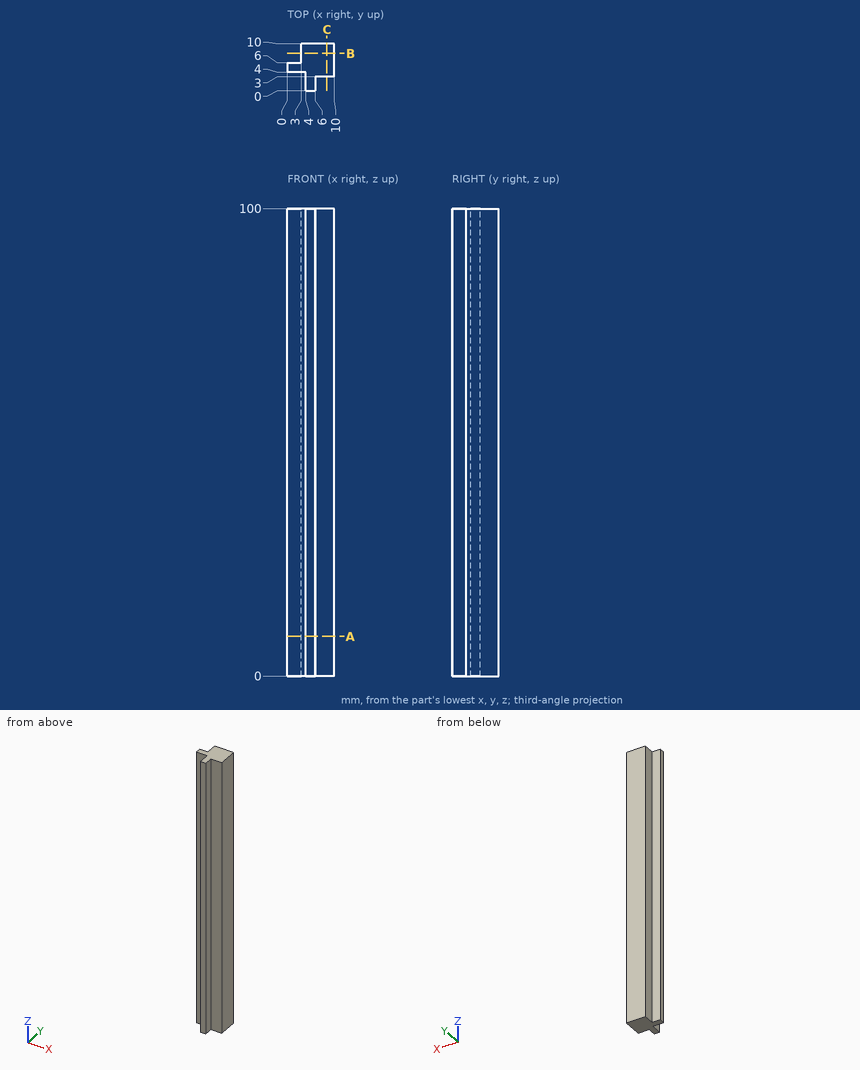
For this review, use the dimensioned drawing (mm, ordinates from the lowest corner) and the shaded views. Round coordinates to 2 decimals unless told otherwise and drop trailing zeros. Order: outer loops, then holes, each group sorted by start corner. A loop starts at its lowest first (then second) coordinate and runs counter-clockwise, first axis right, second up.
1) Consider section A-A (z = 8.5). State the section outline as (x, y) points.
The answers:
outline: (0, 4) - (4, 4) - (4, 0) - (6, 0) - (6, 3) - (10, 3) - (10, 10) - (3, 10) - (3, 6) - (0, 6) - close
2) Clearance check with flat-ended pins moving along their axes: pin 1 Ø1.5 at (x, y) = (3, 5) entering from -Z; pin 2 Ø1.5 at (x, z) = (1, 34.5) entering from +Y. State where each tip first meets the part, or that it passes through.
The answers:
pin 1: stops at z = 0
pin 2: stops at y = 6
3) For L1, parallel to X at y = 2.25, z = 82; L2, parallel to X at y = 9.5, z = 22; L3, parallel to Y at x = 3.25, z = 44.5, list the stretches that pass through material, from the lowest coordinate up.
The answers:
L1: x = 4 to 6
L2: x = 3 to 10
L3: y = 4 to 10
4) Consider section B-B (y = 8). State the section outline as (x, z) points, plus the area to 3 significant figures.
The answers:
outline: (3, 0) - (10, 0) - (10, 100) - (3, 100) - close
area: 700 mm2
